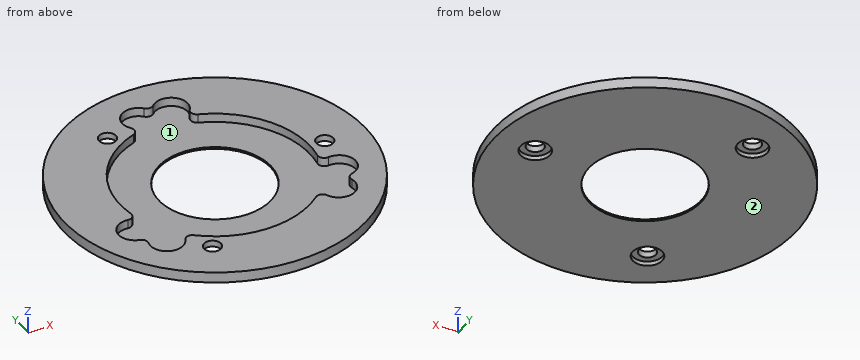
```python
from build123d import *

# Parameters (mm, degrees)
SKETCH_W         = 15.1
SKETCH_H         = 1.7
POCKET_DEPTH     = 5.2
HOLE_D           = 2.7
HOLE_CBORE_D     = 4.7
HOLE_CBORE_DEPTH = 0.7


with BuildPart() as part:
    # Sketch → Revolution (revolve)
    with BuildSketch(Plane.XZ):
        with Locations((16.45, 0.85)):
            Rectangle(SKETCH_W, SKETCH_H)
    revolve(axis=Axis((0, 0, 0), (0, 0, 1)))

    # Sketch001 → Pocket (cut)
    with BuildSketch(Plane.XY.offset(0.3)):
        with BuildLine():
            ThreePointArc((-15.971238, -3.820499), (-18.844764, -5.933151), (-16.905745, -8.926586))
            ThreePointArc((-16.183523, -10.177512), (-16.277605, -9.39788), (-16.905745, -8.926586))
            ThreePointArc((-16.183523, -10.177512), (-14.560642, -13.353469), (-11.294268, -11.921249))
            ThreePointArc((-9.729552, -11.547546), (-10.60619, -11.33964), (-11.294268, -11.921249))
            ThreePointArc((-9.729552, -11.547546), (0, -15.1), (9.729552, -11.547546))
            ThreePointArc((11.294268, -11.921249), (10.60619, -11.33964), (9.729552, -11.547546))
            ThreePointArc((11.294268, -11.921249), (14.560642, -13.353469), (16.183523, -10.177512))
            ThreePointArc((16.905745, -8.926586), (16.277605, -9.39788), (16.183523, -10.177512))
            ThreePointArc((16.905745, -8.926586), (18.844764, -5.933151), (15.971238, -3.820499))
            ThreePointArc((14.865244, -2.652266), (15.123511, -3.51541), (15.971238, -3.820499))
            ThreePointArc((14.865244, -2.652266), (13.076984, 7.55), (5.135693, 14.199812))
            ThreePointArc((4.67697, 15.741748), (4.517321, 14.85505), (5.135693, 14.199812))
            ThreePointArc((4.67697, 15.741748), (4.284123, 19.28662), (0.722222, 19.104098))
            ThreePointArc((-0.722222, 19.104098), (0, 18.795759), (0.722222, 19.104098))
            ThreePointArc((-0.722222, 19.104098), (-4.284123, 19.28662), (-4.67697, 15.741748))
            ThreePointArc((-5.135693, 14.199812), (-4.517321, 14.85505), (-4.67697, 15.741748))
            ThreePointArc((-5.135693, 14.199812), (-13.076984, 7.55), (-14.865244, -2.652266))
            ThreePointArc((-15.971238, -3.820499), (-15.123511, -3.51541), (-14.865244, -2.652266))
        make_face()
    extrude(amount=POCKET_DEPTH, mode=Mode.SUBTRACT)

    # Hole (through all)
    with Locations(Plane(origin=(0, 0, 0), x_dir=(1, 0, 0), z_dir=(0, 0, -1))):
        with Locations((-8.75, -15.155445), (-8.75, 15.155445), (17.5, 0)):
            CounterBoreHole(HOLE_D / 2, HOLE_CBORE_D / 2, HOLE_CBORE_DEPTH)


solid = part.part
```
Check sheet for the modelled part. Datum: model origin and axes. Units: mm. Face numbers are marked on the shaded views. Round coordinates to 2 decimals unless told otherwise and drop trailing zeros. Order: outer loops, then holes, each group sorted by start corner. A loop starts at its lowest first (then second) coordinate and runs counter-clockwise, first axis right, second up. Notation, with made-up numbers: (-24.5, 86.5) -> (6.5, 86.5) arc R18 ccw to (6.5, 93.5) -> close; hole circle Ø4 at (-30.75, -22). An arc over 180 degrees is marked (long way). One line per item, written item: value. Start each with the question number.
Q1. Gauge pin test, flat ends, axial feed: pin 1 Ø3 at (x, y) = (-8.75, 15.16) entering from -Z; pin 2 Ø1 at (y, z) = (-3.5, 1) entering from +X; pin 3 Ø20.5 at (x, y) = (0, 0) entering from +Z. Record the tip position at first contact, or that the pin passes through.
Q2. Cross-section at B-B (y = 0). Record the boundary of the cut face in (x, z), and give its area (3 significant figures).
Q3. Cross-section at D-D (z = 1). Record the boundary of the cut face in (x, y), and give its area (3 significant figures).
Q4. Cross-section at C-C (y = 5). Record the boundary of the cut face in (x, z).
Q5. Mould release check, pull along Y, two halves, no side actions. Record for the marked faces 1 and 2: pulls with the +Y half, pulls with the -Y half, needs draft (parallel to the pull), parting line crosses it, or undercut.
Q6. Cross-section at A-A (x = 0). Record the boundary of the cut face in (y, z), and give its area (3 significant figures).
Q7. Thickness scan on line 1 (X direction, y = 1, z = 0.6); line 2 (X direction, y = -4.5, z = 0.1); line 3 (X direction, y = -3, z = 1.1). Record the ranges inside material, lowest first.
Completed:
1. pin 1: stops at z = 0.7
1. pin 2: stops at x = 23.81
1. pin 3: stops at z = 0.3
2. outline: (-24, 0) -> (-8.9, 0) -> (-8.9, 0.3) -> (-15.1, 0.3) -> (-15.1, 1.7) -> (-24, 1.7) -> close; (8.9, 0) -> (15.15, 0) -> (15.15, 0.7) -> (16.15, 0.7) -> (16.15, 1.7) -> (15.1, 1.7) -> (15.1, 0.3) -> (8.9, 0.3) -> close; (18.85, 0.7) -> (19.85, 0.7) -> (19.85, 0) -> (24, 0) -> (24, 1.7) -> (18.85, 1.7) -> close
2. area: 28.0 mm²
3. outline: circle Ø48 at (0, 0); hole (-16.91, -8.93) arc R1 cw to (-16.18, -10.18) arc R2.6 ccw to (-11.29, -11.92) arc R1 cw to (-9.73, -11.55) arc R15.1 ccw to (9.73, -11.55) arc R1 cw to (11.29, -11.92) arc R2.6 ccw to (16.18, -10.18) arc R1 cw to (16.91, -8.93) arc R2.6 ccw to (15.97, -3.82) arc R1 cw to (14.87, -2.65) arc R15.1 ccw to (5.14, 14.2) arc R1 cw to (4.68, 15.74) arc R2.6 ccw to (0.72, 19.1) arc R1 cw to (-0.72, 19.1) arc R2.6 ccw to (-4.68, 15.74) arc R1 cw to (-5.14, 14.2) arc R15.1 ccw to (-14.87, -2.65) arc R1 cw to (-15.97, -3.82) arc R2.6 ccw to start; hole circle Ø2.7 at (-8.75, -15.16); hole circle Ø2.7 at (-8.75, 15.16); hole circle Ø2.7 at (17.5, 0)
3. area: 940 mm²
4. outline: (-23.47, 0) -> (-7.36, 0) -> (-7.36, 0.3) -> (-14.25, 0.3) -> (-14.25, 1.7) -> (-23.47, 1.7) -> close; (7.36, 0) -> (23.47, 0) -> (23.47, 1.7) -> (14.25, 1.7) -> (14.25, 0.3) -> (7.36, 0.3) -> close
5. face 1: undercut
5. face 2: needs draft
6. outline: (-24, 0) -> (-8.9, 0) -> (-8.9, 0.3) -> (-15.1, 0.3) -> (-15.1, 1.7) -> (-24, 1.7) -> close; (8.9, 0) -> (24, 0) -> (24, 1.7) -> (18.8, 1.7) -> (18.8, 0.3) -> (8.9, 0.3) -> close
6. area: 28.8 mm²
7. line 1: x = -23.98 to -15.07, 15.07 to 15.37, 19.63 to 23.98
7. line 2: x = -23.57 to -7.68, 7.68 to 23.57
7. line 3: x = -23.81 to -14.86, 14.86 to 23.81
